from build123d import *

# Parameters (mm, degrees)
SKETCH1_W                       = 16
SKETCH1_H                       = 8
BOSS_EXTRUDE1_DEPTH             = 3
SHELL1_T                        = -1
SKETCH3_R                       = 1.5
SKETCH3_R_2                     = 0.8
BOSS_EXTRUDE2_DEPTH             = 2
BOSS_EXTRUDE3_DEPTH             = 11
CUT_EXTRUDE1_REACH              = 20.868
SKETCH6_R                       = 1.2
BOSS_EXTRUDE5_DEPTH             = 3.5
BOSS_EXTRUDE5_DIRECTION_2_REACH = 18.513


with BuildPart() as part:
    # Sketch1 → Boss-Extrude1 (new body)
    with BuildSketch(Plane(origin=(0, 0, 0), x_dir=(1, 0, 0), z_dir=(0, 1, 0))):
        Rectangle(SKETCH1_W, SKETCH1_H)
    extrude(amount=BOSS_EXTRUDE1_DEPTH)

    # Shell1
    shell1_openings = [part.faces().sort_by_distance(p)[0] for p in [
        (0, 0, 0),
    ]]
    offset(amount=SHELL1_T, openings=shell1_openings, kind=Kind.INTERSECTION)

    # Sketch3 → Boss-Extrude2 (add)
    with BuildSketch(Plane.XZ.offset(-2)):
        with Locations(Location((0, 0, 0), (0, 0, 270))):
            Circle(SKETCH3_R)
        with Locations(Location((0, 0, 0), (0, 0, 270))):
            Circle(SKETCH3_R_2, mode=Mode.SUBTRACT)
    extrude(amount=BOSS_EXTRUDE2_DEPTH)

    # Sketch4 → Boss-Extrude3 (add)
    with BuildSketch(Plane(origin=(0, 3, 0), x_dir=(1, 0, 0), z_dir=(0, 1, 0))):
        with BuildLine():
            Line((-4, 4), (4, 4))
            Line((4, 4), (4, 2.5))
            Line((4, 2.5), (2, 2.5))
            ThreePointArc((2, 2.5), (0, 1.5), (-2, 2.5))
            Line((-2, 2.5), (-4, 2.5))
            Line((-4, 2.5), (-4, 4))
        make_face()
    extrude(amount=BOSS_EXTRUDE3_DEPTH)

    # Sketch5 → Cut-Extrude1 (cut, up to next)
    with BuildSketch(Plane(origin=(4, 0, 0), x_dir=(0, 0, -1), z_dir=(1, 0, 0)), mode=Mode.PRIVATE) as cut_extrude1_sk1:
        Polygon((3.25, 14), (1.5, 14), (1.5, 10), align=None)
    cut_extrude1_tool1 = extrude(cut_extrude1_sk1.sketch, amount=-CUT_EXTRUDE1_REACH, mode=Mode.PRIVATE) & part.part
    add(cut_extrude1_tool1.solids().sort_by_distance((4, 12.666667, -2.083333))[0], mode=Mode.SUBTRACT)

    # Sketch6 → Boss-Extrude5 (add)
    with BuildSketch(Plane(origin=(0, 1.055737705, 2.413114754), x_dir=(1, 0, 0), z_dir=(0, 0.400818834019708, 0.9161573349021891))):
        with Locations(Location((0, 13.229478025, 0), (0, 0, 270))):
            Circle(SKETCH6_R)
    extrude(amount=BOSS_EXTRUDE5_DEPTH)

    # Sketch6 → Boss-Extrude5 direction 2 (add, up to next)
    with BuildSketch(Plane(origin=(0, 1.055737705, 2.413114754), x_dir=(1, 0, 0), z_dir=(0, 0.400818834019708, 0.9161573349021891)), mode=Mode.PRIVATE) as boss_extrude5_direction_2_sk1:
        with Locations(Location((0, 13.229478025, 0), (0, 0, 270))):
            Circle(SKETCH6_R)
    boss_extrude5_direction_2_tool1 = extrude(boss_extrude5_direction_2_sk1.sketch, amount=-BOSS_EXTRUDE5_DIRECTION_2_REACH, mode=Mode.PRIVATE) - part.part
    add(boss_extrude5_direction_2_tool1.solids().sort_by_distance((0, 13.176021, -2.889509))[0])


solid = part.part
The model under review builds one solid part; all positions refer to its coordinate system, in mm. A direction names the side the tool comes from. Coordinates: 2 decimals unless noted, no trailing zeros. Write each loop counter-clockwise with the first axis right and the second up, starting at its lowest first coordinate (ties: lowest second). Pieces come first, ordered by that corner, then holes. Notation, with made-up numbers: (-25.75, 3.5) -> (5.25, 3.5) arc R16 cw to (5.25, 15.5) -> close; hole circle Ø8 at (25.5, 15). An arc over 180 degrees is marked (long way). Answer in a Markdown table with one row per item.
1. We need section A-A, the plane x = 4.25. State the section outline as (y, z) points, and give its area (3 significant figures).
Answers below:
| item | result |
|---|---|
| outline | (0, -4) -> (3, -4) -> (3, 4) -> (0, 4) -> (0, 3) -> (2, 3) -> (2, -3) -> (0, -3) -> close |
| area | 12.0 mm^2 |
2. Draft analysis for pull direction X (two halves, no side actions). For faces 1 (the flat face through (0, 1, 3)), 2 (the flat face through (3, 8, -2.5)), 3 (the flat face through (8, 1, 0)), 4 (the flat face through (-8, 1, 0)), state which applies: +X half, -X half, draft (parallel to the pull), parting line (faces both ways), or undercut.
Answers below:
| item | result |
|---|---|
| face 1 | undercut |
| face 2 | draft |
| face 3 | +X half |
| face 4 | -X half |
3. We need section D-D, the plane y = 10.75. State the section outline as (x, z) points.
Answers below:
| item | result |
|---|---|
| outline | (-4, -4) -> (4, -4) -> (4, -2.5) -> (2, -2.5) arc R2.5 ccw to (1.24, -1.83) -> (-1.24, -1.83) arc R2.5 ccw to (-2, -2.5) -> (-4, -2.5) -> close |
4. Clearance check with flat-ended pins moving along their axes: pin 1 Ø0.6 at (x, z) = (2, -4) entering from +Y; pin 2 Ø4 at (y, z) = (13, -1) entering from +X; pin 3 Ø2 at (x, y) = (4, 11) entering from +Z. State where each tip first meets the part, or that it passes through.
Answers below:
| item | result |
|---|---|
| pin 1 | stops at y = 14 |
| pin 2 | stops at x = 4 |
| pin 3 | stops at z = -2.5 |
5. We need section C-C, the plane z = 1.25. State the section outline as (x, y) points.
Answers below:
| item | result |
|---|---|
| outline | (-8, 0) -> (-7, 0) -> (-7, 2) -> (-0.83, 2) -> (-0.83, 0) -> (0.83, 0) -> (0.83, 2) -> (7, 2) -> (7, 0) -> (8, 0) -> (8, 3) -> (-8, 3) -> close |
6. For faces 5 (the flat face through (-3, 8, -2.5)), 6 (the flat face through (-7, 1, 0)), 7 (the cylindrical face through (0, 6.5, -1.5)), 8 (the flat face through (4, 8, -3)), list the 3-axis set-ups (+Z, -Z, +X, -X, +Y, -Y) from which the entire face can be reached by the end or side of a thin tool; tool diameter is ignored.
Answers below:
| item | result |
|---|---|
| face 5 | +Z, -X, +Y |
| face 6 | -Y |
| face 7 | +Z |
| face 8 | +Z, -Z, +X, +Y |
7. Wall thickness on probe 1 along X at (y, z) = (0.7, 0); probe 2 along X at (y, z) = (7.5, -2.75); probe 3 along Y at (x, z) = (2.5, 0): over which ranges is each line inside the solid? List them lowest first. Write a range as [from, to].
Answers below:
| item | result |
|---|---|
| probe 1 | x = [-8, -7], [-1.5, -0.8], [0.8, 1.5], [7, 8] |
| probe 2 | x = [-4, 4] |
| probe 3 | y = [2, 3] |
8. We need section B-B, the plane y = 7.5. State the section outline as (x, z) points.
Answers below:
| item | result |
|---|---|
| outline | (-4, -4) -> (4, -4) -> (4, -2.5) -> (2, -2.5) arc R2.5 ccw to (-2, -2.5) -> (-4, -2.5) -> close |
